Geometry: see drawing. Coordinates: mm, zero at the bounding-box minimum. Round coordinates to 2 decimals unless told otherwise and drop trailing zeros. Loops run counter-clockwise (first coordinate to the right, second up) from the corner with the lowest first, then second, coordinate; pieces in that order, holes last.
(1) Cut plane B-B, the plane y = 20. Output: boundary loops of the cut face in (x, z).
(2) Cut plane C-C, the plane z = 80.5. Output: boundary loops of the cut face in (x, y), and give its area (3 significant figures).
(3) Draft query along X for the marked faces 1, 2 and 3. Return one class per face: released by +X, released by -X, zero draft, split by the parting line, or undercut.
(4) Cut plane D-D, the plane y = 9. Output: boundary loops of the cut face in (x, z).
(5) First-contact query: pin 1 Ø3.5 at (y, z) = (32, 65) entering from +X; pin 2 Ø4 at (x, z) = (33, 62) entering from -Y; pin 3 Ø8 at (y, z) = (7, 81) entering from +X. Flat tips, straight axial feed; report the tip coordinate or a pass-through.
(6) Line query: line 1 (Y direction, x = 20, z = 78); line 2 (X direction, y = 20.5, z = 47.5); line 3 (X direction, y = 12, z = 41). Output: solid intervals per line, ascending.
(7) Cut plane A-A, the plane x = 20. Output: boundary loops of the cut face in (y, z), and give its area (3 significant figures).
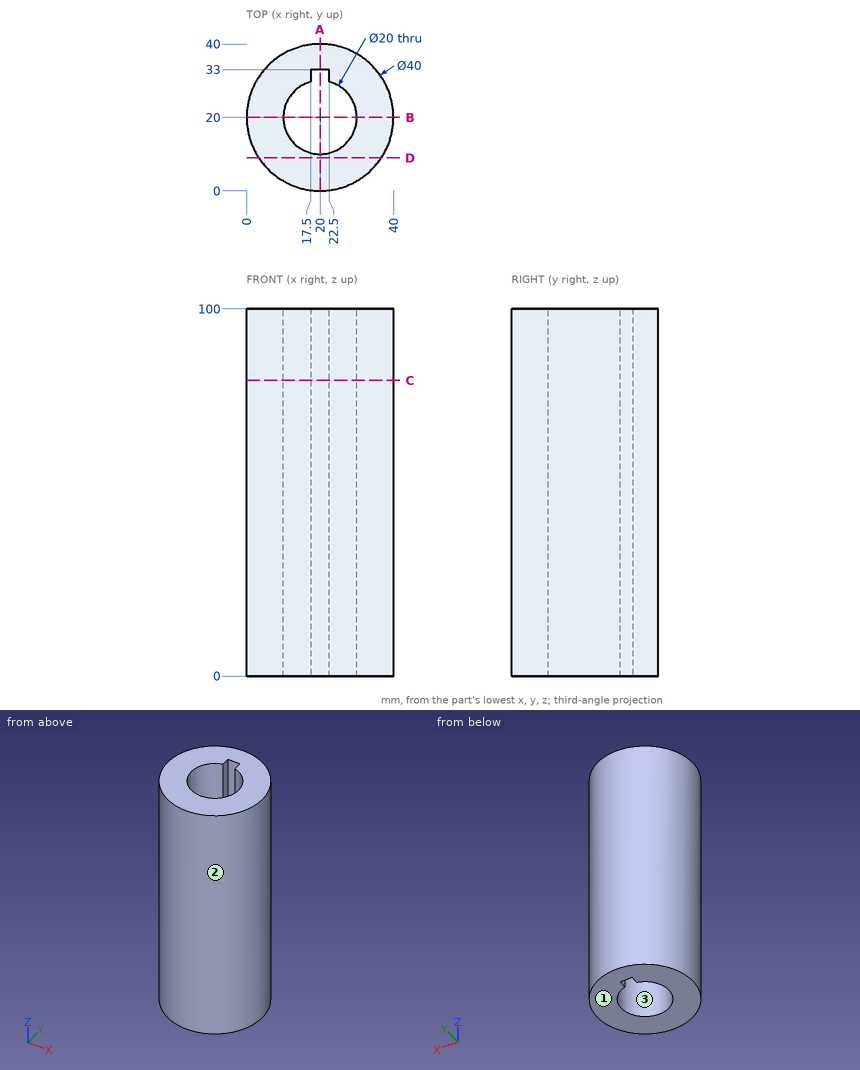
Reported:
1. outline: (0, 0) - (10, 0) - (10, 100) - (0, 100) - close; (30, 0) - (40, 0) - (40, 100) - (30, 100) - close
2. outline: circle Ø40 at (20, 20); hole (17.5, 29.68) arc R10 ccw (long way) to (22.5, 29.68) - (22.5, 33) - (17.5, 33) - close
2. area: 927 mm2
3. face 1: zero draft
3. face 2: split by the parting line
3. face 3: undercut
4. outline: (3.3, 0) - (36.7, 0) - (36.7, 100) - (3.3, 100) - close
5. pin 1: stops at x = 37.17
5. pin 2: stops at y = 3.3
5. pin 3: stops at x = 37.86
6. line 1: y = 0 to 10, 33 to 40
6. line 2: x = 0.01 to 10.01, 29.99 to 39.99
6. line 3: x = 1.67 to 14, 26 to 38.33
7. outline: (0, 0) - (10, 0) - (10, 100) - (0, 100) - close; (33, 0) - (40, 0) - (40, 100) - (33, 100) - close
7. area: 1,700 mm2
